Verification items for this drawing (mm, ordinates from the low corner). Give positions to 0.01 mm unless a question says otherwise; leave off trailing zeros. Loops run counter-clockwise (first coordinate to the right, second up) from the corner with the lowest first, then second, coordinate; pieces in that order, holes last. Notation, with made-up numbers: M -7,-37 L 45,-37 A24 ccw 45,-27 Z; hole C 69,-36.75 d11. An arc over 180 degrees is marked long. Answer in a Markdown table with one row per item.
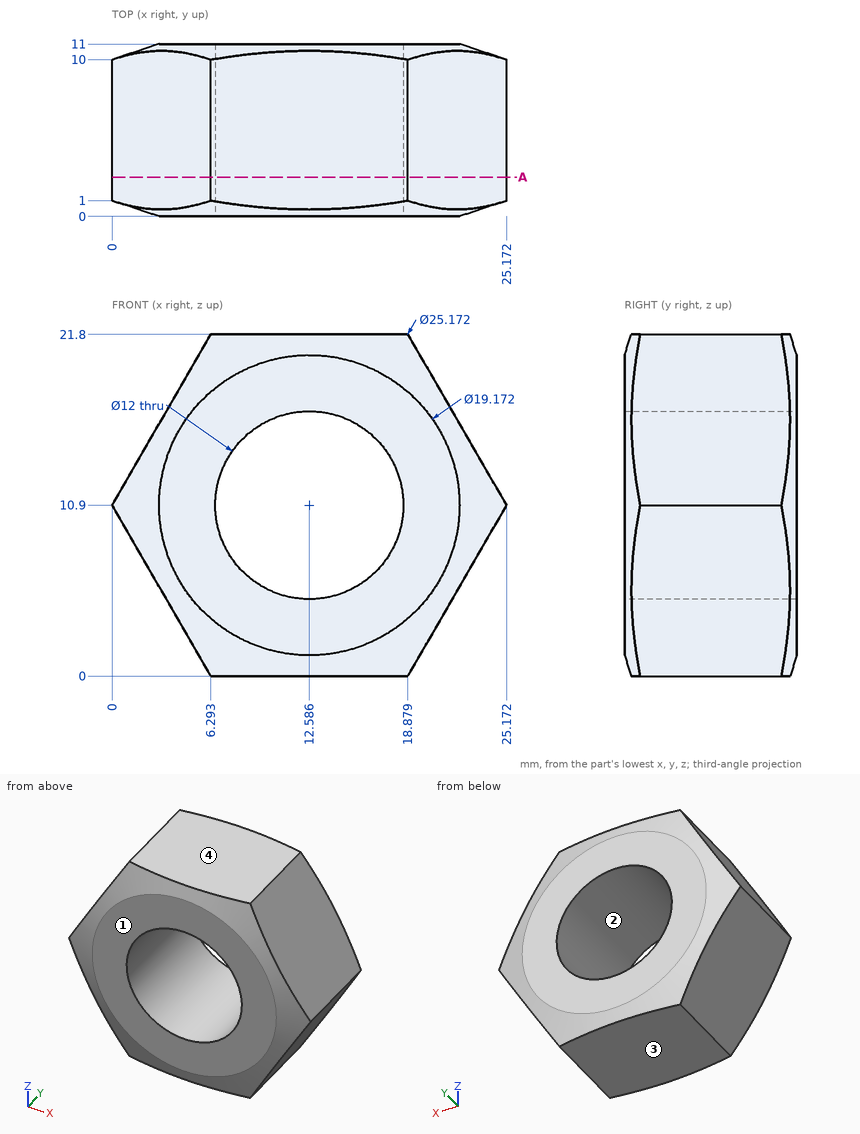
Item 1: Scan lines: L1, parallel to X at y = 3, z = 8 (1 decimal); L2, parallel to Z at x = 7.75, y = 7.5; L3, parallel to Z at x = 16.75, y = 0.75. Record each from-to range of solid material in increasing order. Write a range as [from, to].
Reported:
| item | result |
|---|---|
| L1 | x = [1.7, 7.3], [17.8, 23.5] |
| L2 | z = [0, 7.35], [14.45, 21.8] |
| L3 | z = [0, 6.58], [15.22, 21.8] |
Item 2: Go/stop test with flat-tipped pins: pin 1 (8 mm diameter, centred on x = 20.5, z = 5, fed in from +Y); pin 2 (1 mm diameter, centred on y = 2.5, z = 3, fed in from -X); pin 3 (5 mm diameter, centred on y = 1, z = 13.5, fed in from +X) (1 decimal). Record where each tip stops, or that it passes through.
Reported:
| item | result |
|---|---|
| pin 1 | stops at y = 11 |
| pin 2 | stops at x = 4.27 |
| pin 3 | stops at x = 25.1 |
Item 3: Release check for a two-part mould opening along Z. For the marked faces 1, 2, 3 and 4 record: released by +Z, released by -Z, zero draft, split by the parting line, or undercut.
Reported:
| item | result |
|---|---|
| face 1 | zero draft |
| face 2 | undercut |
| face 3 | released by -Z |
| face 4 | released by +Z |
Item 4: Sectioned sample at A-A (y = 2.5). Record the cut outline in (x, z).
Reported:
| item | result |
|---|---|
| outline | M 0,10.9 L 6.29,0 L 18.88,0 L 25.17,10.9 L 18.88,21.8 L 6.29,21.8 Z; hole C 12.59,10.9 d12 |
